For this review, take the finished solid that the model builds, in its own axes (mm). Face numbers are marked on the shaded views. A direction names the side the tool comes from. Give positions to 0.01 mm unless a question says otherwise; leave off trailing zeros. Loops run counter-clockwise (first coordinate to the right, second up) from the corner with the lowest first, then second, coordinate; pieces in that order, holes last. Notation, with made-up numbers: (36, 27.5) - (51, 27.5) arc R13 cw to (51, 46.5) - close; hole circle Ø7 at (76, 3). An arc over 180 degrees is marked (long way). Put each result on its own line as item: value.
from build123d import *

# Parameters (mm, degrees)
F0_W        = 1300
F0_H        = 900
F1_DEPTH    = 35
F2_W        = 125
F2_H        = 500
F3_DEPTH    = 75
F4_R        = 40
F5_R        = 40
F6_DEPTH    = 625
F7_W        = 125
F7_H        = 800
F7_R        = 40
F8_DEPTH    = 25
F9_T1_DEPTH = 341.5063509461
F9_T3_DEPTH = 341.5063509461


# Not quite as in the source:
# - a fillet or chamfer that OpenCascade refuses, or shapes differently, is made with other operations: its cross-section is extruded or revolved along the edge and cut away or added


with BuildPart() as f1:
    # F0 (on Top) → F1 (new body)
    with BuildSketch(Plane.XY):
        with Locations((-10.7608698308, 73.6055876629)):
            Rectangle(F0_W, F0_H)
    extrude(amount=F1_DEPTH)

    # F2 (on face) → F3 (join)
    with BuildSketch(Plane(origin=(0, 0, 0), x_dir=(1, 0, 0), z_dir=(0, 0, -1))):
        with Locations((-448.2608698308, -73.6055876629)):
            Rectangle(F2_W, F2_H)
        with Locations((426.7391301692, -73.6055876629)):
            Rectangle(F2_W, F2_H)
    extrude(amount=F3_DEPTH)

    # F4 (on face) + F5 (on face) → F6 (join)
    with BuildSketch(Plane(origin=(0, 0, -75), x_dir=(1, 0, 0), z_dir=(0, 0, -1))):
        with Locations((-448.2608698308, -73.6055876629)):
            Circle(F4_R)
    with BuildSketch(Plane(origin=(0, 0, -75), x_dir=(1, 0, 0), z_dir=(0, 0, -1))):
        with Locations((426.7391301692, -73.6055876629)):
            Circle(F5_R)
    extrude(amount=F6_DEPTH)

    # F7 (on face) → F8 (join)
    with BuildSketch(Plane(origin=(0, 0, -700), x_dir=(1, 0, 0), z_dir=(0, 0, -1))):
        with Locations((-448.2608698308, -73.6055876629)):
            Rectangle(F7_W, F7_H)
        with Locations((-448.2608698308, -73.6055876629)):
            Circle(F7_R, mode=Mode.SUBTRACT)
        with Locations((426.7391301692, -73.6055876629)):
            Rectangle(F7_W, F7_H)
        with Locations((-448.2608698308, -73.6055876629)):
            Circle(F7_R)
    extrude(amount=F8_DEPTH)

    # F9: fillet of radius 50 on 4 edges, made by hand

    # F9_s2 → F9_t1 (cut)
    with BuildSketch(Plane.YZ.offset(-619.0140453039)):
        with BuildLine():
            ThreePointArc((-283.0931421479, -700), (-308.0931421479, -706.6987298108), (-326.3944123371, -725))
            Line((-326.3944123371, -725), (-326.3944123371, -700))
            Line((-326.3944123371, -700), (-283.0931421479, -700))
        make_face()
        with BuildLine():
            ThreePointArc((430.3043174737, -700), (455.3043174737, -706.6987298108), (473.6055876629, -725))
            Line((473.6055876629, -725), (473.6055876629, -700))
            Line((473.6055876629, -700), (430.3043174737, -700))
        make_face()
    extrude(amount=F9_T1_DEPTH, mode=Mode.SUBTRACT)

    # F9_s4 → F9_t3 (cut)
    with BuildSketch(Plane.YZ.offset(255.9859546961)):
        with BuildLine():
            ThreePointArc((-326.3944123371, -725), (-308.0931421479, -706.6987298108), (-283.0931421479, -700))
            Line((-283.0931421479, -700), (-326.3944123371, -700))
            Line((-326.3944123371, -700), (-326.3944123371, -725))
        make_face()
        with BuildLine():
            ThreePointArc((473.6055876629, -725), (455.3043174737, -706.6987298108), (430.3043174737, -700))
            Line((430.3043174737, -700), (473.6055876629, -700))
            Line((473.6055876629, -700), (473.6055876629, -725))
        make_face()
    extrude(amount=F9_T3_DEPTH, mode=Mode.SUBTRACT)


solid = f1.part
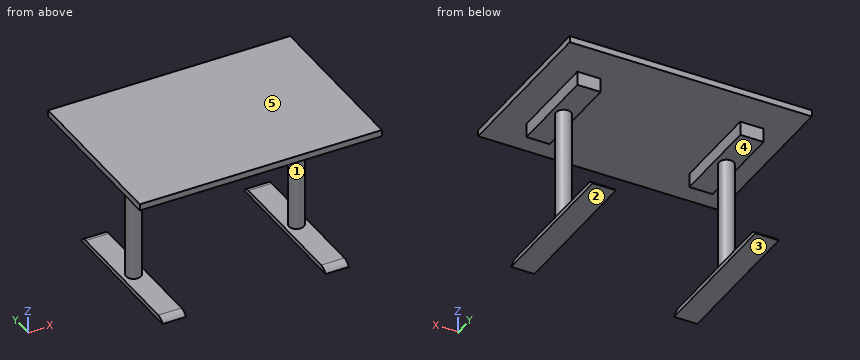
1) Take a section at C-C on y = 180.5. State the section outline as (x, z) points, and give its area (3 significant figures).
Geometry check:
outline: (-660.76, 0) - (-510.76, 0) - (-510.76, -75) - (-385.76, -75) - (-385.76, 0) - (364.24, 0) - (364.24, -75) - (489.24, -75) - (489.24, 0) - (639.24, 0) - (639.24, 35) - (-660.76, 35) - close; (-510.76, -725) - (-385.76, -725) - (-385.76, -700) - (-510.76, -700) - close; (364.24, -725) - (489.24, -725) - (489.24, -700) - (364.24, -700) - close
area: 70,500 mm²
2) Take a section at D-D on x = 523. State the section outline as (y, z) points, and give its area (3 significant figures).
Geometry check:
outline: (-376.39, 0) - (523.61, 0) - (523.61, 35) - (-376.39, 35) - close
area: 31,500 mm²
3) For the marked faces 1 and 2, list the 3-axis set-ups (+Z, -Z, +X, -X, +Y, -Y) from which the entire face can be reached by the end or side of a thin tool; tool diameter is ignored.
Geometry check:
face 1: none
face 2: -Z, +X, -X, +Y, -Y
4) Insertion check: pin 1 Ø22.5 at (x, z) = (443.5, -53) entering from +Y; pin 2 Ø22.5 at (x, z) = (-426.5, -34) entering from -Y; pin 3 Ø20 at (y, z) = (-111, -718.5) entering from +X. Each pin has a flat end and moves straight along its axis. Give the tip position at first contact, or say it passes through.
Geometry check:
pin 1: stops at y = 323.61
pin 2: stops at y = -176.39
pin 3: stops at x = 489.24
5) Draft analysis for pull direction Z (two halves, no side actions). For the marked faces 3, 4 and 5, state which applies: pulls with the +Z half, pulls with the -Z half, needs draft (parallel to the pull), parting line crosses it, or undercut.
Geometry check:
face 3: pulls with the -Z half
face 4: undercut
face 5: pulls with the +Z half
6) Wall thickness on line 1 (Z direction, x = 477, y = 435); line 2 (Z direction, x = 482, y = -37); line 3 (Z direction, x = 512.5, y = -282): over which ranges is each line inside the solid? List them lowest first.
Geometry check:
line 1: z = -725 to -700.22, 0 to 35
line 2: z = -725 to -700, -75 to 35
line 3: z = 0 to 35
7) Take a section at A-A on y = -197. State the section outline as (x, z) points, and give its area (4 significant figures).
Geometry check:
outline: (-660.76, 0) - (639.24, 0) - (639.24, 35) - (-660.76, 35) - close; (-510.76, -725) - (-385.76, -725) - (-385.76, -700) - (-510.76, -700) - close; (364.24, -725) - (489.24, -725) - (489.24, -700) - (364.24, -700) - close
area: 51,750 mm²
8) Take a section at B-B on z = -28. State the section outline as (x, y) points.
Geometry check:
outline: (-510.76, -176.39) - (-385.76, -176.39) - (-385.76, 323.61) - (-510.76, 323.61) - close; (364.24, -176.39) - (489.24, -176.39) - (489.24, 323.61) - (364.24, 323.61) - close
